```python
from build123d import *

# Parameters (mm, degrees)
SKETCH1_R               = 10.85
BOSS_EXTRUDE1_DEPTH     = 1
SKETCH2_W               = 1
SKETCH2_H               = 1
BOSS_EXTRUDE2_DEPTH     = 4.4
CIRPATTERN1_COUNT       = 2
SKETCH3_R               = 10.85
SKETCH3_R_2             = 10.35
BOSS_EXTRUDE3_DEPTH     = 6.3
CUT_EXTRUDE1_DEPTH      = 1.8
CUT_EXTRUDE4_DEPTH      = 2.8
CUT_EXTRUDE4_DEPTH_BACK = 2.5
BOSS_EXTRUDE4_DEPTH     = 7.3


with BuildPart() as part:
    # Sketch1 → Boss-Extrude1 (new body)
    with BuildSketch(Plane(origin=(0, 0, 0), x_dir=(1, 0, 0), z_dir=(0, 1, 0))):
        Circle(SKETCH1_R)
    extrude(amount=BOSS_EXTRUDE1_DEPTH)

    # Sketch2 → Boss-Extrude2 (add)
    with BuildSketch(Plane.XZ):
        with Locations((0, 9)):
            Rectangle(SKETCH2_W, SKETCH2_H)
    boss_extrude2 = extrude(amount=BOSS_EXTRUDE2_DEPTH)

    # CirPattern1: Boss-Extrude2 ×2 about axis
    cirpattern1_axis = Axis((0, 0, 0), (0, 1, 0))
    for i in range(1, CIRPATTERN1_COUNT):
        add(boss_extrude2.rotate(cirpattern1_axis, i * 360 / CIRPATTERN1_COUNT))

    # Sketch3 → Boss-Extrude3 (add)
    with BuildSketch(Plane(origin=(0, 1, 0), x_dir=(1, 0, 0), z_dir=(0, 1, 0))):
        Circle(SKETCH3_R)
        Circle(SKETCH3_R_2, mode=Mode.SUBTRACT)
    extrude(amount=BOSS_EXTRUDE3_DEPTH)

    # Sketch4 → Cut-Extrude1 (cut)
    with BuildSketch(Plane(origin=(0, 7.3, 0), x_dir=(1, 0, 0), z_dir=(0, 1, 0))):
        with BuildLine():
            Line((-3.75, 9.646761114), (-3.75, 10.181355509))
            ThreePointArc((-3.75, 10.181355509), (0, -10.85), (3.75, 10.181355509))
            Line((3.75, 10.181355509), (3.75, 9.646761114))
            ThreePointArc((3.75, 9.646761114), (0, -10.35), (-3.75, 9.646761114))
        make_face()
    extrude(amount=-CUT_EXTRUDE1_DEPTH, mode=Mode.SUBTRACT)

    # Sketch7 → Cut-Extrude4 (cut, two sides)
    with BuildSketch(Plane(origin=(0, 5.5, 0), x_dir=(1, 0, 0), z_dir=(0, 1, 0))) as cut_extrude4_sk:
        with BuildLine():
            Line((-6.5, -8.687491007), (-6.5, -8.054346653))
            ThreePointArc((-6.5, -8.054346653), (-10.227312895, 1.58888985), (-3.75, 9.646761114))
            Line((-3.75, 9.646761114), (-3.75, 10.181355509))
            ThreePointArc((-3.75, 10.181355509), (-10.736571483, 1.56477883), (-6.5, -8.687491007))
        make_face()
        with BuildLine():
            Line((6.5, -8.687491007), (6.5, -8.054346653))
            ThreePointArc((6.5, -8.054346653), (10.227312895, 1.58888985), (3.75, 9.646761114))
            Line((3.75, 9.646761114), (3.75, 10.181355509))
            ThreePointArc((3.75, 10.181355509), (10.736571483, 1.56477883), (6.5, -8.687491007))
        make_face()
    extrude(amount=CUT_EXTRUDE4_DEPTH, mode=Mode.SUBTRACT)
    extrude(cut_extrude4_sk.sketch, amount=-CUT_EXTRUDE4_DEPTH_BACK, mode=Mode.SUBTRACT)

    # Sketch8 → Boss-Extrude4 (add)
    with BuildSketch(Plane.XZ):
        with BuildLine():
            Line((-3.75, -10.181355509), (-3.75, -14.85))
            Line((-3.75, -14.85), (3.75, -14.85))
            Line((3.75, -14.85), (3.75, -10.181355509))
            ThreePointArc((3.75, -10.181355509), (0, -10.85), (-3.75, -10.181355509))
        make_face()
    extrude(amount=-BOSS_EXTRUDE4_DEPTH)


solid = part.part
```
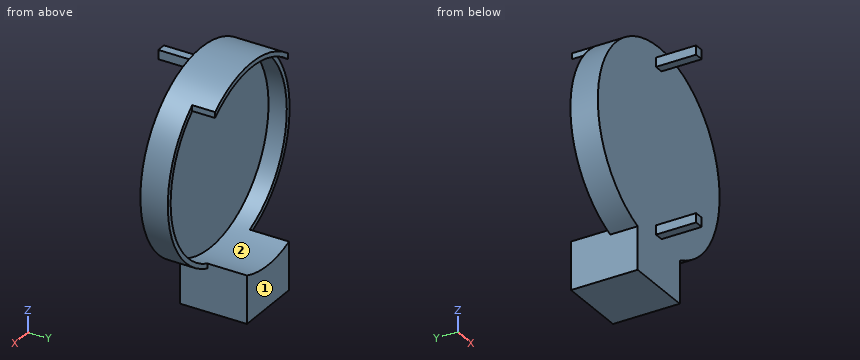
Geometry: final body of the model. Coordinates: model frame, mm. Face numbers are marked on the shaded views. A direction names the side the tool comes from. Coordinates: 2 decimals unless noted, no trailing zeros. Order: outer loops, then holes, each group sorted by start corner. A loop starts at its lowest first (then second) coordinate and runs counter-clockwise, first axis right, second up.
Item 1: Access query for the marked faces 1 and 2. Directions: +Z, -Z, +X, -X, +Y, -Y. A direction counts if a zero-diameter tool reaches every point of the face in a straight line with its end or side. Return the directions, or none.
Answer:
face 1: +Z, -Z, +X, -X, +Y
face 2: +Y
Item 2: Contact query for flat-ended pins moving along their axis: P1, Ø2, axis at y = -2.5, z = -11.5, coming from the -X side; P2, Ø1.1, axis at y = -1.5, z = -9, coming from the +X side; P3, Ø4, axis at x = -5, z = 0.5, coming from the -Y side; P4, Ø0.8, axis at x = 0, y = -2, coming from the +Z side. Output: stop coordinate, or through.
Answer:
P1: passes through
P2: stops at x = 0.5
P3: stops at y = 0
P4: stops at z = 9.5
Item 3: Section query D-D (y = -0.5). Output: boundary loops of the cut face in (x, z), then the cut area to 3 significant figures.
Answer:
outline: (-0.5, -9.5) - (0.5, -9.5) - (0.5, -8.5) - (-0.5, -8.5) - close; (-0.5, 8.5) - (0.5, 8.5) - (0.5, 9.5) - (-0.5, 9.5) - close
area: 2.00 mm2
Item 4: Material intervals for line 1 along Z through (x, y) = (0, 3.5); line 2 along X through (y, z) = (2.5, 0); line 3 along Z through (x, y) = (0, 6), sorted ascending.
Answer:
line 1: z = -14.85 to -10.35, 10.35 to 10.85
line 2: x = -10.85 to -10.35, 10.35 to 10.85
line 3: z = -14.85 to -10.35
Item 5: Section query C-C (z = 0). Output: boundary loops of the cut face in (x, y), then the cut area to 3 significant figures.
Answer:
outline: (-10.85, 0) - (10.85, 0) - (10.85, 3) - (10.35, 3) - (10.35, 1) - (-10.35, 1) - (-10.35, 3) - (-10.85, 3) - close
area: 23.7 mm2
Item 6: Section query B-B (x = 0). Output: boundary loops of the cut face in (y, z).
Answer:
outline: (-4.4, -9.5) - (0, -9.5) - (0, -14.85) - (7.3, -14.85) - (7.3, -10.35) - (1, -10.35) - (1, 10.35) - (5.5, 10.35) - (5.5, 10.85) - (0, 10.85) - (0, 9.5) - (-4.4, 9.5) - (-4.4, 8.5) - (0, 8.5) - (0, -8.5) - (-4.4, -8.5) - close
Item 7: Section query A-A (y = 4.75). Output: boundary loops of the cut face in (x, z), then the cut area to 3 significant figures.
Answer:
outline: (-6.5, 8.05) arc R10.35 cw to (6.5, 8.05) - (6.5, 8.69) arc R10.85 ccw to (-6.5, 8.69) - close; (-3.75, -14.85) - (3.75, -14.85) - (3.75, -9.65) arc R10.35 cw to (-3.75, -9.65) - close
area: 42.5 mm2
